The model under review builds one solid part; all positions refer to its coordinate system, in mm. Face numbers are marked on the shaded views. A direction names the side the tool comes from. Round coordinates to 2 decimals unless told otherwise and drop trailing zeros. Write each loop counter-clockwise with the first axis right and the second up, starting at its lowest first coordinate (ties: lowest second). Pieces come first, ordered by that corner, then holes. Notation, with made-up numbers: (81, 23.5) -> (129, 23.5) arc R25 ccw to (129, 56.5) -> close; hole circle Ø1 at (77, -29.75). An arc over 180 degrees is marked (long way). Return JSON: item names as keys, results as strings. Group by question number.
1. Take a section at A-A, the plane y = -28.5. Write out the cut boundary in (x, z), then the cut area to 3 significant figures.
2. Take a section at B-B, the plane x = 0. Give the number of separate pieces and of enclosed holes in the cut face, then the cut area to 3 significant figures.
3. Tool access review of the marked faces 3 and 4: name each direction out of +Z, -Z, +X, -X, +Y, -Y from which nothing blocks a thin tool from reaching the whole face with its end or side.
4. For line 1 along Z through (x, y) = (16, -22); line 2 along Z through (x, y) = (-9, 4.5) (3 decimals); line 3 along X through (y, z) = (-1, 9), list the stretches that pass through material, from the lowest coordinate up. Write a range as from..to.
5. Mouldability with a two-part tool opening along X and no side actions: class the marked faces 1 and 2 as pulls with the +X half, pulls with the -X half, needs draft (parallel to the pull), parting line crosses it, or undercut.
6. Take a section at D-D, the plane y = 5. Write out the cut boundary in (x, z) (1 decimal).
7. Clearance check with flat-ended pins moving along their axes: P1, Ø4, axis at x = -16, z = -11.5, coming from the +Y side; P2, Ø12, axis at x = -17, y = -22.5, coming from the +Z side; P3, Ø5, axis at x = 7, y = 6, coming from the -Z side; P4, Ø6, axis at y = -23, z = -16.5, coming from the +X side. State where each tip first meets the part, or that it passes through.
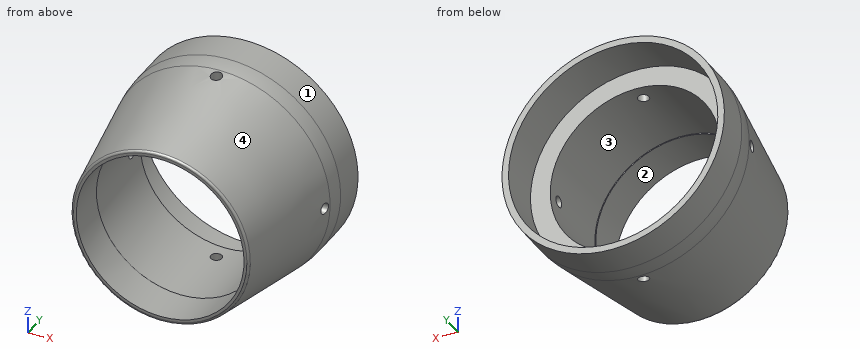
from build123d import *

# Parameters (mm, degrees)
F_6_40_TAPPED_HOLE1_REACH  = 74.325
F_6_40_TAPPED_HOLE1_BORE_R = 1.4351
CIRPATTERN1_COUNT          = 4
FILLET1_R                  = 0.635
FILLET2_R                  = 25.4


with BuildPart() as part:
    # Sketch2 → Revolve1 (revolve)
    with BuildSketch(Plane.XY, mode=Mode.PRIVATE) as revolve1_sk:
        Polygon((22.0472, -22.4282), (22.0472, -0.0762), (27.1907, -0.0762), (27.1907, 10.922), (28.8925, 10.922), (28.8925, -0.0762), (23.0632, -32.512), (21.7932, -32.512), (21.7932, -22.4282), align=None)
    revolve(revolve1_sk.sketch.rotate(Axis((0, -34.5451, 0), (0, 1, 0)), 90), axis=Axis((0, -34.5451, 0), (0, 1, 0)))

    # #6-40 Tapped Hole1 bore → #6-40 Tapped Hole1 (cut, up to next)
    with BuildSketch(Plane.XY.offset(28.8925), mode=Mode.PRIVATE) as f_6_40_tapped_hole1_sk1:
        with Locations((0, -4.318)):
            Circle(F_6_40_TAPPED_HOLE1_BORE_R)
    f_6_40_tapped_hole1_tool1 = extrude(f_6_40_tapped_hole1_sk1.sketch, amount=-F_6_40_TAPPED_HOLE1_REACH, mode=Mode.PRIVATE) & part.part
    f_6_40_tapped_hole1 = f_6_40_tapped_hole1_tool1.solids().sort_by_distance((0, -4.318, 28.8925))[0]
    add(f_6_40_tapped_hole1, mode=Mode.SUBTRACT)

    # CirPattern1: #6-40 Tapped Hole1 ×4 about axis
    cirpattern1_axis = Axis((0, -34.5451, 0), (0, -1, 0))
    for i in range(1, CIRPATTERN1_COUNT):
        add(f_6_40_tapped_hole1.rotate(cirpattern1_axis, i * 360 / CIRPATTERN1_COUNT), mode=Mode.SUBTRACT)

    # Fillet1
    fillet1_edges = [part.edges().sort_by_distance(p)[0] for p in [
        (0, -32.512, 23.0632),
    ]]
    fillet(fillet1_edges, radius=FILLET1_R)

    # Fillet2
    fillet2_edges = [part.edges().sort_by_distance(p)[0] for p in [
        (0, -0.0762, 28.8925),
    ]]
    fillet(fillet2_edges, radius=FILLET2_R)


solid = part.part
Output:
{
 "1": {"outline": "circle Ø47.57 at (0, 0); hole circle Ø43.59 at (0, 0)", "area": "285 mm^2"},
 "2": {"separate pieces": "4", "enclosed holes": "0", "area": "262 mm^2"},
 "3": {"face 3": "+Y", "face 4": "-Y"},
 "4": {"line 1": "z = -19.15..-15.17, 15.17..19.15", "line 2": "z = -27.455..-25.658, 25.658..27.455", "line 3": "x = -27.24..-20.13, 20.13..27.24"},
 "5": {"face 1": "parting line crosses it", "face 2": "undercut"},
 "6": {"outline": "circle Ø57.8 at (0, 0); hole circle Ø54.4 at (0, 0)"},
 "7": {"P1": "passes through", "P2": "stops at z = 22.53", "P3": "stops at z = -28.54", "P4": "stops at x = 20.87"}
}
